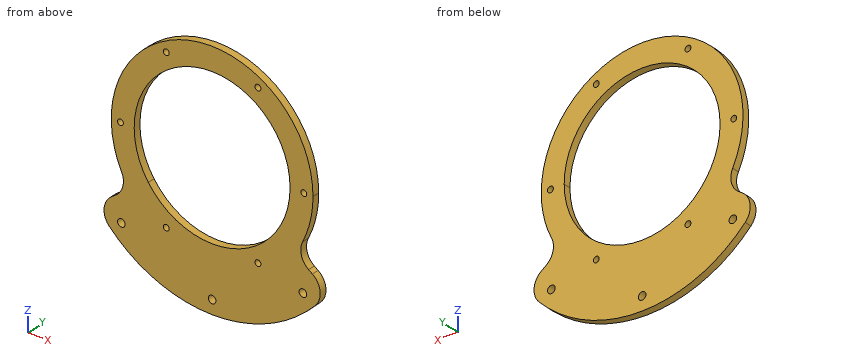
from build123d import *

# Parameters (mm, degrees)
SKETCH_1_R      = 2.075
SKETCH_1_R_2    = 1.6
EXTRUDE_1_DEPTH = 4
FILLET_1_R      = 10


with BuildPart() as part:
    # 草图1 → 凸台-拉伸1 (new body)
    # profile 1 of 3: a face of its own
    with BuildSketch(Plane(origin=(0, 0, 0), x_dir=(1, 0, 0), z_dir=(0, 1, 0))):
        with BuildLine():
            Line((-63.484283432, 44.452173817), (-45.053362436, 31.546703999))
            ThreePointArc((-45.053362436, 31.546703999), (0, 55), (45.053362436, 31.546703999))
            Line((45.053362436, 31.546703999), (63.484283432, 44.452173817))
            ThreePointArc((63.484283432, 44.452173817), (0, 77.5), (-63.484283432, 44.452173817))
        make_face()
        with Locations(Location((-49.497474683, 49.497474683, 0), (0, 0, 270))):
            Circle(SKETCH_1_R, mode=Mode.SUBTRACT)
        with Locations(Location((0, 70, 0), (0, 0, 270))):
            Circle(SKETCH_1_R, mode=Mode.SUBTRACT)
        with Locations(Location((49.497474683, 49.497474683, 0), (0, 0, 270))):
            Circle(SKETCH_1_R, mode=Mode.SUBTRACT)
    # profile 2 of 3: a face of its own
    with BuildSketch(Plane(origin=(0, 0, 0), x_dir=(1, 0, 0), z_dir=(0, 1, 0))):
        with BuildLine():
            Line((-45.053362436, 31.546703999), (-34.813961882, 24.376998545))
            ThreePointArc((-34.813961882, 24.376998545), (0, 42.5), (34.813961882, 24.376998545))
            Line((34.813961882, 24.376998545), (45.053362436, 31.546703999))
            ThreePointArc((45.053362436, 31.546703999), (0, 55), (-45.053362436, 31.546703999))
        make_face()
        with Locations(Location((-25, 43.301270189, 0), (0, 0, 270))):
            Circle(SKETCH_1_R_2, mode=Mode.SUBTRACT)
        with Locations(Location((25, 43.301270189, 0), (0, 0, 270))):
            Circle(SKETCH_1_R_2, mode=Mode.SUBTRACT)
    # profile 3 of 3: a face of its own
    with BuildSketch(Plane(origin=(0, 0, 0), x_dir=(1, 0, 0), z_dir=(0, 1, 0))):
        with BuildLine():
            ThreePointArc((42.5, 0), (-12.779996479, -40.532970407), (-34.813961882, 24.376998545))
            Line((-34.813961882, 24.376998545), (-45.053362436, 31.546703999))
            ThreePointArc((-45.053362436, 31.546703999), (-16.538818973, -52.454432291), (55, 0))
            ThreePointArc((55, 0), (52.454432291, 16.538818973), (45.053362436, 31.546703999))
            Line((45.053362436, 31.546703999), (34.813961882, 24.376998545))
            ThreePointArc((34.813961882, 24.376998545), (40.532970407, 12.779996479), (42.5, 0))
        make_face()
        with Locations(Location((-25, -43.301270189, 0), (0, 0, 270))):
            Circle(SKETCH_1_R_2, mode=Mode.SUBTRACT)
        with Locations(Location((-50, 0, 0), (0, 0, 270))):
            Circle(SKETCH_1_R_2, mode=Mode.SUBTRACT)
        with Locations(Location((25, -43.301270189, 0), (0, 0, 270))):
            Circle(SKETCH_1_R_2, mode=Mode.SUBTRACT)
        with Locations(Location((50, 0, 0), (0, 0, 270))):
            Circle(SKETCH_1_R_2, mode=Mode.SUBTRACT)
    extrude(amount=EXTRUDE_1_DEPTH)

    # 圆角1
    fillet_1_edges = [part.edges().sort_by_distance(p)[0] for p in [
        (-45.053362436, 2, -31.546703999),
        (-63.484283432, 2, -44.452173817),
        (63.484283432, 2, -44.452173817),
        (45.053362436, 2, -31.546703999),
    ]]
    fillet(fillet_1_edges, radius=FILLET_1_R)


solid = part.part
The listing builds one solid part. Answer for the finished solid, in the listing's coordinates (mm). Round coordinates to 2 decimals unless told otherwise and drop trailing zeros. Loops run counter-clockwise (first coordinate to the right, second up) from the corner with the lowest first, then second, coordinate; pieces in that order, holes last. Notation, with made-up numbers: M 34.5,35 L 82.5,35 A19 ccw 82.5,48 Z; hole C 32.5,-34 d3. An arc over 180 degrees is marked long. Write each question's results on one line, items separated by ' | '. Start each with the question number.
1) Find section B-B on z = -70. Write down the section's boundary in (x, y) (3 decimals).
2) Find section A-A on x = 0. Write down the section's boundary in (y, z) (3 decimals), plus the area to 3 significant figures.
3) Each of these flat-tipped pins is pushed along its axis until it touches: pin 1 (1.9 mm diameter, centred on x = 25, z = -43.3, fed in from +Y); pin 2 (1.5 mm diameter, centred on y = 1, z = -13.5, fed in from +X); pin 3 (1 mm diameter, centred on x = 47, y = 1, fed in from -Z). Where does it stop, or does it pass through?
4) Find section D-D on y = 1.25. Count the separate pieces of the cut face and the enclosed holes in it, plus the area to 3 significant figures.
5) Find section C-C on x = 16. Write down the section's boundary in (y, z).
6) Straight lines are drawn through the part: probe 1 along Z at (x, y) = (50.5, 3.65); probe 2 along X at (y, z) = (0.95, 39); probe 3 along X at (y, z) = (0.9, -9.5). For each, find the intervals that lie inside material, in ascending order.
Final values:
1) outline: M -33.26,0 L -2.075,0 L -2.075,4 L -33.26,4 Z; M 2.075,0 L 33.26,0 L 33.26,4 L 2.075,4 Z
2) outline: M 0,-77.5 L 4,-77.5 L 4,-72.075 L 0,-72.075 Z; M 0,-67.925 L 4,-67.925 L 4,-42.5 L 0,-42.5 Z; M 0,42.5 L 4,42.5 L 4,55 L 0,55 Z | area: 173 mm²
3) pin 1: through | pin 2: x = 53.5 | pin 3: z = -62
4) separate pieces: 1 | enclosed holes: 10 | area: 6,580 mm²
5) outline: M 0,-75.83 L 4,-75.83 L 4,-39.37 L 0,-39.37 Z; M 0,39.37 L 4,39.37 L 4,52.62 L 0,52.62 Z
6) probe 1: -58.79 to -51.31, -47.68 to -34.85, -21.79 to -1.52, 1.52 to 21.79 | probe 2: -38.78 to -16.89, 16.89 to 38.78 | probe 3: -54.17 to -41.42, 41.42 to 54.17
